Input: part model. Units: mm. Frame: model coordinates. A direction names the side the tool comes from. Round coordinates to 2 decimals unless told otherwise and drop trailing zeros. Order: outer loops, then holes, each group sorted by start corner. A loop starts at its lowest first (then second) coordinate and runs counter-clockwise, first axis right, second up. Notation, with made-up numbers: (65, 54.5) -> (71, 54.5) arc R22 cw to (71, 93.5) -> close; hole circle Ø7 at (85, 59.5). An arc over 180 degrees is marked (long way). Answer as CSV lines item,"result". Start each with the question number.
1) Line query: L1, parallel to Y at x = 38.1, z = 2.1 (3 decimals); L2, parallel to Y at x = 14, z = 0.55; L3, parallel to X at y = -2.5, z = 5.05. Output: solid intervals per line, ascending.
2) Mould query, pull axis X, two halves, no side actions, for faces 5 (the face through (-10.36, -8.496, 2.962)), 6 (the face through (48, 22.225, 3)), 7 (the face through (50.8, -21, 3)). Classes: +X half, -X half, draft (parallel to the pull), parting line (faces both ways), or undercut.
3) First-contact query: P1, Ø1, axis at x = -2.5, z = 4.5, coming from the +Y side; P2, Ø4, axis at x = 38.1, y = 6.35, coming from the +Z side; P3, Ø1, axis at y = 20.5, z = 2.5, coming from the +X side; P4, Ø1.6, axis at y = 21.5, z = 3.5, coming from the -X side. Flat tips, straight axial feed; report the tip coordinate or a pass-through.
4) Section query B-B, the plane z = 4.6. State how many separate pieces and enclosed holes the cut face has, and give its area (3 significant figures).
5) Access query for faces 1 (the face through (-54, 19.05, 3)), 2 (the face through (54, 19.05, 3)), 3 (the face through (-54, -19.05, 3)), 4 (the face through (-54, -6.35, 3)). Directions: +Z, -Z, +X, -X, +Y, -Y. A direction counts if a zero-diameter tool reaches every point of the face in a straight line with its end or side. Return the directions, or none.
6) Section query A-A, the plane x = -12.7. Output: boundary loops of the cut face in (y, z) (3 decimals), and give its area (3 significant figures).
```python
from build123d import *

# Parameters (mm, degrees)
BOSS_EXTRUDE1_DEPTH = 5.842
FILLET1_R           = 1.5875
SKETCH2_R           = 3.175
CUT_EXTRUDE1_DEPTH  = 62.126064432


with BuildPart() as part:
    # Sketch1 → Boss-Extrude1 (new body)
    with BuildSketch(Plane.XY):
        Polygon((50.8, -22.225), (44.45, -22.225), (44.45, -19.05), (-44.45, -19.05), (-44.45, -22.225), (-50.8, -22.225), (-50.8, -19.05), (-56.642, -19.05), (-56.642, -6.35), (-50.8, -6.35), (-50.8, 6.35), (-56.642, 6.35), (-56.642, 19.05), (-50.8, 19.05), (-50.8, 22.225), (-44.45, 22.225), (-44.45, 19.05), (44.45, 19.05), (44.45, 22.225), (50.8, 22.225), (50.8, 19.05), (56.642, 19.05), (56.642, 6.35), (50.8, 6.35), (50.8, -6.35), (56.642, -6.35), (56.642, -19.05), (50.8, -19.05), align=None)
    extrude(amount=BOSS_EXTRUDE1_DEPTH)

    # Fillet1
    fillet1_edges = [part.edges().sort_by_distance(p)[0] for p in [
        (-44.45, -19.05, 2.921),
        (44.45, -19.05, 2.921),
        (44.45, 19.05, 2.921),
        (-44.45, 19.05, 2.921),
    ]]
    fillet(fillet1_edges, radius=FILLET1_R)
    fillet1_2_edges = [part.edges().sort_by_distance(p)[0] for p in [
        (-44.45, -22.225, 2.921),
        (44.45, -22.225, 2.921),
        (44.45, 22.225, 2.921),
        (-44.45, 22.225, 2.921),
    ]]
    fillet(fillet1_2_edges, radius=FILLET1_R - 0.0001)  # a hair under: the kernel refuses the full size

    # Sketch2 → Cut-Extrude1 (cut, through all)
    with BuildSketch(Plane.XY.offset(5.842)):
        with Locations((-38.1, 6.35)):
            Circle(SKETCH2_R)
        with Locations((-12.7, 6.35)):
            Circle(SKETCH2_R)
        with Locations(Location((-12.7, -6.35, 0), (0, 0, 180))):
            Circle(SKETCH2_R)
        with Locations(Location((-38.1, -6.35, 0), (0, 0, 180))):
            Circle(SKETCH2_R)
        with Locations((38.1, -6.35)):
            Circle(SKETCH2_R)
        with Locations((12.7, -6.35)):
            Circle(SKETCH2_R)
        with Locations(Location((12.7, 6.35, 0), (0, 0, 180))):
            Circle(SKETCH2_R)
        with Locations(Location((38.1, 6.35, 0), (0, 0, 180))):
            Circle(SKETCH2_R)
    extrude(amount=-CUT_EXTRUDE1_DEPTH, mode=Mode.SUBTRACT)


solid = part.part
```
Findings:
1,L1,"y = -19.05 to -9.525, -3.175 to 3.175, 9.525 to 19.05"
1,L2,"y = -19.05 to -9.25, -3.45 to 3.45, 9.25 to 19.05"
1,L3,"x = -50.8 to 50.8"
2,face 5,"undercut"
2,face 6,"draft"
2,face 7,"+X half"
3,P1,"stops at y = 19.05"
3,P2,"passes through"
3,P3,"stops at x = 50.8"
3,P4,"stops at x = -50.8"
4,separate pieces,"1"
4,enclosed holes,"8"
4,area,"4,000 mm^2"
5,face 1,"+Z, -Z, -X, +Y"
5,face 2,"+Z, -Z, +X, +Y"
5,face 3,"+Z, -Z, -X, -Y"
5,face 4,"+Z, -Z, -X"
6,outline,"(-19.05, 0) -> (-9.525, 0) -> (-9.525, 5.842) -> (-19.05, 5.842) -> close; (-3.175, 0) -> (3.175, 0) -> (3.175, 5.842) -> (-3.175, 5.842) -> close; (9.525, 0) -> (19.05, 0) -> (19.05, 5.842) -> (9.525, 5.842) -> close"
6,area,"148 mm^2"
